Geometry: final body of the model. Coordinates: model frame, mm. A direction names the side the tool comes from. Round coordinates to 2 decimals unless told otherwise and drop trailing zeros. Write each loop counter-clockwise with the first axis right and the second up, starting at its lowest first coordinate (ties: lowest second). Pieces come first, ordered by that corner, then holes. Notation, with made-up numbers: (48, 36.5) -> (95, 36.5) arc R33 ccw to (95, 75.5) -> close; hole circle Ø10 at (57.25, 24). An arc over 180 degrees is marked (long way). One line per item, written item: value. Start each with the question number.
from build123d import *

# Parameters (mm, degrees)
ESQUISSE2_W             = 70
ESQUISSE2_H             = 55
BOSS_EXTRU_1_DEPTH      = 2
ESQUISSE3_W             = 13
ESQUISSE3_H             = 9
BOSS_EXTRU_2_DEPTH      = 10
ESQUISSE4_W             = 38.871257781
ESQUISSE4_H             = 1.325156515
ESQUISSE4_W_2           = 50.503187194
ESQUISSE4_H_2           = 1.251536709
BOSS_EXTRU_3_DEPTH      = 6
ESQUISSE5_R             = 1.5
ENL_V_MAT_EXTRU_1_DEPTH = 6
ESQUISSE6_R             = 1.5
ENL_V_MAT_EXTRU_2_DEPTH = 6


with BuildPart() as part:
    # Esquisse2 → Boss.-Extru.1 (new body)
    with BuildSketch(Plane(origin=(0, 0, 0), x_dir=(1, 0, 0), z_dir=(0, 1, 0))):
        Rectangle(ESQUISSE2_W, ESQUISSE2_H)
    extrude(amount=BOSS_EXTRU_1_DEPTH)

    # Esquisse3 → Boss.-Extru.2 (add)
    with BuildSketch(Plane(origin=(0, 2, 0), x_dir=(1, 0, 0), z_dir=(0, 1, 0))):
        with Locations((28.5, 18)):
            Rectangle(ESQUISSE3_W, ESQUISSE3_H)
    extrude(amount=BOSS_EXTRU_2_DEPTH)

    # Esquisse4 → Boss.-Extru.3 (add)
    with BuildSketch(Plane(origin=(0, 2, 0), x_dir=(1, 0, 0), z_dir=(0, 1, 0))):
        with Locations((-13.177945346, 25.325213404)):
            Rectangle(ESQUISSE4_W, ESQUISSE4_H)
        with Locations((-8.024558898, -24.993924275)):
            Rectangle(ESQUISSE4_W_2, ESQUISSE4_H_2)
    extrude(amount=BOSS_EXTRU_3_DEPTH)

    # Esquisse5 → Enlèv. mat.-Extru.1 (cut)
    with BuildSketch(Plane(origin=(0, 2, 0), x_dir=(1, 0, 0), z_dir=(0, 1, 0))):
        with Locations(Location((20, -24.5, 0), (0, 0, 270))):
            Circle(ESQUISSE5_R)
    extrude(amount=-ENL_V_MAT_EXTRU_1_DEPTH, mode=Mode.SUBTRACT)

    # Esquisse6 → Enlèv. mat.-Extru.2 (cut)
    with BuildSketch(Plane(origin=(0, 2, 0), x_dir=(1, 0, 0), z_dir=(0, 1, 0))):
        with Locations(Location((20.7, 24.5, 0), (0, 0, 270))):
            Circle(ESQUISSE6_R)
    extrude(amount=-ENL_V_MAT_EXTRU_2_DEPTH, mode=Mode.SUBTRACT)


solid = part.part
(1) Section query B-B (x = -12). Output: boundary loops of the cut face in (y, z), and give its area (3 significant figures).
(2) Pull-direction query (Z, two-part tool) for faces 1 (the face through (0, 1, -27.5)), 2 (the face through (0, 1, 27.5)), 3 (the face through (-8, 5, 24.368)); classes: pulls with the +Z half, pulls with the -Z half, needs draft (parallel to the pull), parting line crosses it, or undercut.
(3) Line query: probe 1 along X at (y, z) = (0.9, 24.5); probe 2 along X at (y, z) = (0.5, -24.5); probe 3 along Z at (x, y) = (-5, 5). Output: solid intervals per line, ascending.
(4) Section query C-C (x = 29). Output: boundary loops of the cut face in (y, z).
(5) Section query A-A (y = 3). Output: boundary loops of the cut face in (x, z).
(6) Set-up query: faces 4 (the face through (28, 12, -18)), 5 (the face through (-8, 5, 25.62)), 6 (the face through (22, 7, -18)), 7 (the face through (28, 7, -22.5)), 8 (the face through (-13, 5, -24.663)). Return all of +Z, -Z, +X, -X, +Y, -Y with unobstructed straight access to the full face (end or side cutting, diameter ignored); none if empty.
(7) Pin query (flat end, axial travel): pin 1 (5 mm diameter, centred on x = 13.5, z = 2.5, fed in from +Y); pin 2 (6.5 mm diameter, centred on x = 4, y = 4, fed in from +Z); pin 3 (0.7 mm diameter, centred on y = 4.5, z = -25.5, fed in from +X); pin 4 (1.5 mm diameter, centred on y = 4, z = -25.5, fed in from -X). Return the tip coordinate at first contact, or that it passes through.
(8) Section query D-D (y = 10). Output: boundary loops of the cut face in (x, z), and give its area (3 significant figures).
Results list:
1. outline: (0, -27.5) -> (2, -27.5) -> (2, -25.99) -> (8, -25.99) -> (8, -24.66) -> (2, -24.66) -> (2, 24.37) -> (8, 24.37) -> (8, 25.62) -> (2, 25.62) -> (2, 27.5) -> (0, 27.5) -> close
1. area: 125 mm^2
2. face 1: pulls with the -Z half
2. face 2: pulls with the +Z half
2. face 3: undercut
3. probe 1: x = -35 to 18.5, 21.5 to 35
3. probe 2: x = -35 to 19.2, 22.2 to 35
3. probe 3: z = -25.99 to -24.66, 24.37 to 25.62
4. outline: (0, -27.5) -> (2, -27.5) -> (2, -22.5) -> (12, -22.5) -> (12, -13.5) -> (2, -13.5) -> (2, 27.5) -> (0, 27.5) -> close
5. outline: (-33.28, 24.37) -> (17.23, 24.37) -> (17.23, 25.62) -> (-33.28, 25.62) -> close; (-32.61, -25.99) -> (6.26, -25.99) -> (6.26, -24.66) -> (-32.61, -24.66) -> close; (22, -22.5) -> (35, -22.5) -> (35, -13.5) -> (22, -13.5) -> close
6. face 4: +Z, -Z, +X, -X, +Y
6. face 5: +Z, +X, -X, +Y
6. face 6: +Z, -Z, -X, +Y
6. face 7: -Z, +X, -X, +Y
6. face 8: +X, -X, +Y
7. pin 1: stops at y = 2
7. pin 2: stops at z = 27.5
7. pin 3: stops at x = 6.26
7. pin 4: stops at x = -32.61
8. outline: (22, -22.5) -> (35, -22.5) -> (35, -13.5) -> (22, -13.5) -> close
8. area: 117 mm^2
